CAD build for the part. Positions are in the model's coordinates, mm. A direction names the side the tool comes from. Round coordinates to 2 decimals unless told otherwise and drop trailing zeros. Use one line per item in the form item = value.
from build123d import *

# Parameters (mm, degrees)
SKETCH1_R           = 2.5
BOSS_EXTRUDE1_DEPTH = 315.81


with BuildPart() as part:
    # Sketch1 → Boss-Extrude1 (new body)
    with BuildSketch(Plane.XY):
        with BuildLine():
            Line((-31.376404226, -0.06181021), (-29.676404226, -0.06181021))
            ThreePointArc((-29.676404226, -0.06181021), (-29.570338208, -0.017876227), (-29.526404226, 0.08818979))
            Line((-29.526404226, 0.08818979), (-29.526404226, 3.524374304))
            ThreePointArc((-29.526404226, 3.524374304), (-29.43420518, 3.662790523), (-29.27095023, 3.631048831))
            Line((-29.27095023, 3.631048831), (-25.480107929, -0.116419988))
            Line((-25.480107929, -0.116419988), (-25.480107929, -6.007200432))
            Line((-25.480107929, -6.007200432), (-29.27095023, -9.754669251))
            ThreePointArc((-29.27095023, -9.754669251), (-29.43420518, -9.786410942), (-29.526404226, -9.647994723))
            Line((-29.526404226, -9.647994723), (-29.526404226, -6.21181021))
            ThreePointArc((-29.526404226, -6.21181021), (-29.570338208, -6.105744193), (-29.676404226, -6.06181021))
            Line((-29.676404226, -6.06181021), (-31.376404226, -6.06181021))
            ThreePointArc((-31.376404226, -6.06181021), (-31.482470243, -6.105744193), (-31.526404226, -6.21181021))
            Line((-31.526404226, -6.21181021), (-31.526404226, -12.71181021))
            ThreePointArc((-31.526404226, -12.71181021), (-31.423891599, -12.959297583), (-31.176404226, -13.06181021))
            Line((-31.176404226, -13.06181021), (-24.676404226, -13.06181021))
            ThreePointArc((-24.676404226, -13.06181021), (-24.570338208, -13.017876227), (-24.526404226, -12.91181021))
            Line((-24.526404226, -12.91181021), (-24.526404226, -11.21181021))
            ThreePointArc((-24.526404226, -11.21181021), (-24.570338208, -11.105744193), (-24.676404226, -11.06181021))
            Line((-24.676404226, -11.06181021), (-28.094489023, -11.06181021))
            ThreePointArc((-28.094489023, -11.06181021), (-28.233235517, -10.96881381), (-28.199943018, -10.805135682))
            Line((-28.199943018, -10.805135682), (-24.41329202, -7.06181021))
            Line((-24.41329202, -7.06181021), (-18.546923839, -7.06181021))
            Line((-18.546923839, -7.06181021), (-14.760272841, -10.805135682))
            ThreePointArc((-14.760272841, -10.805135682), (-14.726980342, -10.96881381), (-14.865726836, -11.06181021))
            Line((-14.865726836, -11.06181021), (-18.283811633, -11.06181021))
            ThreePointArc((-18.283811633, -11.06181021), (-18.38987765, -11.105744193), (-18.433811633, -11.21181021))
            Line((-18.433811633, -11.21181021), (-18.433811633, -12.91181021))
            ThreePointArc((-18.433811633, -12.91181021), (-18.38987765, -13.017876227), (-18.283811633, -13.06181021))
            Line((-18.283811633, -13.06181021), (-11.783811633, -13.06181021))
            ThreePointArc((-11.783811633, -13.06181021), (-11.53632426, -12.959297583), (-11.433811633, -12.71181021))
            Line((-11.433811633, -12.71181021), (-11.433811633, -6.21181021))
            ThreePointArc((-11.433811633, -6.21181021), (-11.477745616, -6.105744193), (-11.583811633, -6.06181021))
            Line((-11.583811633, -6.06181021), (-13.283811633, -6.06181021))
            ThreePointArc((-13.283811633, -6.06181021), (-13.38987765, -6.105744193), (-13.433811633, -6.21181021))
            Line((-13.433811633, -6.21181021), (-13.433811633, -9.647994723))
            ThreePointArc((-13.433811633, -9.647994723), (-13.526010678, -9.786410942), (-13.689265628, -9.754669251))
            Line((-13.689265628, -9.754669251), (-17.480107929, -6.007200432))
            Line((-17.480107929, -6.007200432), (-17.480107929, -0.116419988))
            Line((-17.480107929, -0.116419988), (-13.689265628, 3.631048831))
            ThreePointArc((-13.689265628, 3.631048831), (-13.526010678, 3.662790523), (-13.433811633, 3.524374304))
            Line((-13.433811633, 3.524374304), (-13.433811633, 0.08818979))
            ThreePointArc((-13.433811633, 0.08818979), (-13.38987765, -0.017876227), (-13.283811633, -0.06181021))
            Line((-13.283811633, -0.06181021), (-11.583811633, -0.06181021))
            ThreePointArc((-11.583811633, -0.06181021), (-11.477745616, -0.017876227), (-11.433811633, 0.08818979))
            Line((-11.433811633, 0.08818979), (-11.433811633, 6.58818979))
            ThreePointArc((-11.433811633, 6.58818979), (-11.53632426, 6.835677164), (-11.783811633, 6.93818979))
            Line((-11.783811633, 6.93818979), (-18.283811633, 6.93818979))
            ThreePointArc((-18.283811633, 6.93818979), (-18.38987765, 6.894255807), (-18.433811633, 6.78818979))
            Line((-18.433811633, 6.78818979), (-18.433811633, 5.08818979))
            ThreePointArc((-18.433811633, 5.08818979), (-18.38987765, 4.982123773), (-18.283811633, 4.93818979))
            Line((-18.283811633, 4.93818979), (-14.865726836, 4.93818979))
            ThreePointArc((-14.865726836, 4.93818979), (-14.726980342, 4.84519339), (-14.760272841, 4.681515262))
            Line((-14.760272841, 4.681515262), (-18.546923839, 0.93818979))
            Line((-18.546923839, 0.93818979), (-24.41329202, 0.93818979))
            Line((-24.41329202, 0.93818979), (-28.199943018, 4.681515262))
            ThreePointArc((-28.199943018, 4.681515262), (-28.233235517, 4.84519339), (-28.094489023, 4.93818979))
            Line((-28.094489023, 4.93818979), (-24.676404226, 4.93818979))
            ThreePointArc((-24.676404226, 4.93818979), (-24.570338208, 4.982123773), (-24.526404226, 5.08818979))
            Line((-24.526404226, 5.08818979), (-24.526404226, 6.78818979))
            ThreePointArc((-24.526404226, 6.78818979), (-24.570338208, 6.894255807), (-24.676404226, 6.93818979))
            Line((-24.676404226, 6.93818979), (-31.176404226, 6.93818979))
            ThreePointArc((-31.176404226, 6.93818979), (-31.423891599, 6.835677164), (-31.526404226, 6.58818979))
            Line((-31.526404226, 6.58818979), (-31.526404226, 0.08818979))
            ThreePointArc((-31.526404226, 0.08818979), (-31.482470243, -0.017876227), (-31.376404226, -0.06181021))
        make_face()
        with Locations(Location((-21.480107929, -3.06181021, 0), (0, 0, 180))):
            Circle(SKETCH1_R, mode=Mode.SUBTRACT)
    extrude(amount=BOSS_EXTRUDE1_DEPTH)


solid = part.part
1. Drop a flat-ended pin along its axis: P1, Ø3, axis at x = -21.5, z = 176.5, coming from the +Y side. Give the stop position or say it passes through.
Completed:
P1 = 0.94
2. Tool access for faces 5 (the face through (-25.48, -3, 156)), 6 (the face through (-21, 0.938, 156)), 7 (the face through (-17.48, -3, 156)): list every direction of +Z, -Z, +X, -X, +Y, -Y with a clear straight run to the whole face (end or side of a thin tool).
Completed:
face_5 = +Z, -Z, -X
face_6 = +Z, -Z, +Y
face_7 = +Z, -Z, +X
3. Probe line 1 along X through (y, z) = (-8.75, 181.5); line 2 along Y through (x, z) = (-30.25, 300); line 3 along X through (y, z) = (5.25, 274.5). List the from-to ranges inside material, lowest first. Write a range as from..to.
Completed:
line_1 = -31.53..-29.53, -28.25..-26.12, -16.84..-14.71, -13.43..-11.43
line_2 = -13.06..-6.06, -0.06..6.94
line_3 = -31.53..-24.53, -18.43..-11.43
4. Pull direction X, two halves, no side cores. Call faces 1 (the face through (-22, -7.062, 156)), 2 (the face through (-31.526, -9, 156)), 3 (the face through (-11.434, 3, 156)), 4 (the face through (-19, -1, 315.81)): +X half, -X half, draft (parallel to the pull), parting line (faces both ways), or undercut.
Completed:
face_1 = undercut
face_2 = -X half
face_3 = +X half
face_4 = draft
